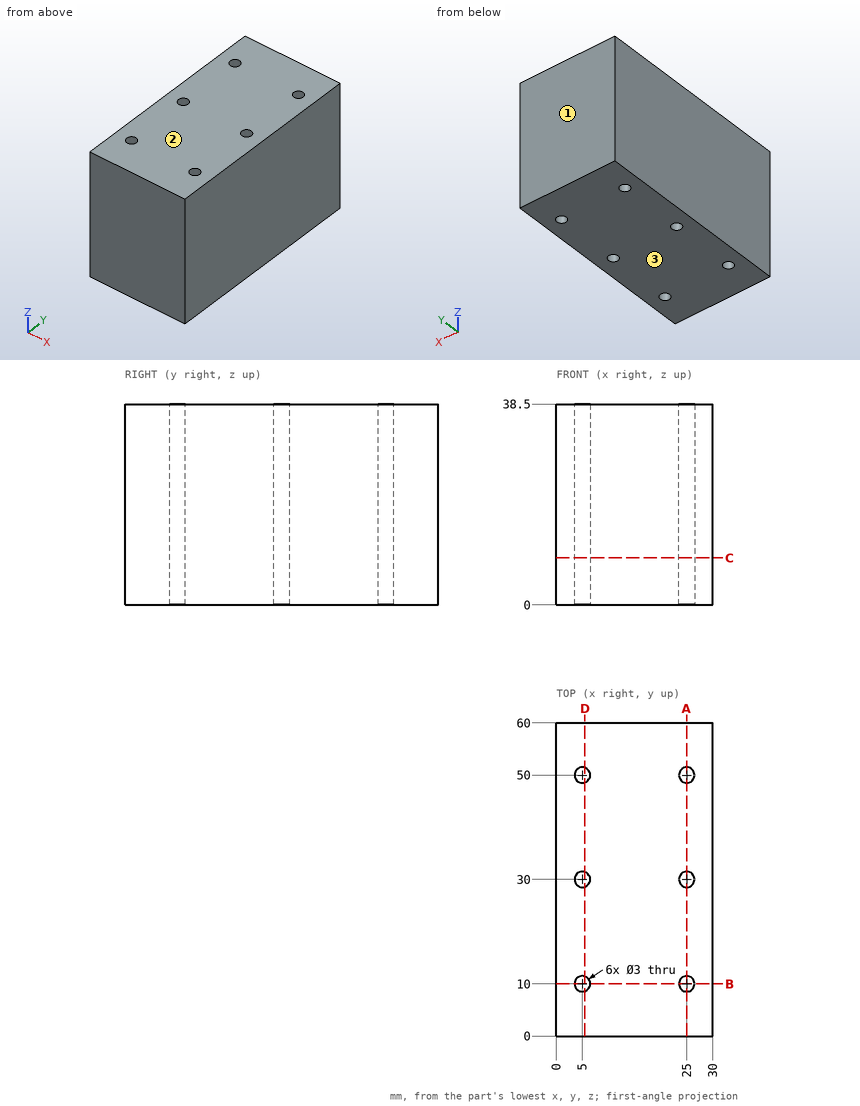
Can you work these out from the drawing? Everything is in mm from the part's minimum corner. Give positions to 0.01 mm unless a question says otherwise; leave off trailing zeros. Order: outer loops, then holes, each group sorted by start corner. A loop starts at its lowest first (then second) coordinate and runs counter-clockwise, first axis right, second up. Notation, with made-up numbers: M 30.25,8.5 L 88.25,8.5 A12 cw 88.25,25.5 Z; hole C -6.75,27.25 d9. An arc over 180 degrees is marked long. One line per question, with ' | ' between items.
1. I want a section at A-A (x = 25). List the corners of the cut face in (y, z) for me, and give its area (3 significant figures).
Results:
outline: M 0,0 L 8.5,0 L 8.5,38.5 L 0,38.5 Z; M 11.5,0 L 28.5,0 L 28.5,38.5 L 11.5,38.5 Z; M 31.5,0 L 48.5,0 L 48.5,38.5 L 31.5,38.5 Z; M 51.5,0 L 60,0 L 60,38.5 L 51.5,38.5 Z | area: 1,960 mm²
2. I want a section at D-D (x = 5.5). List the corners of the cut face in (y, z) for me.
Results:
outline: M 0,0 L 8.59,0 L 8.59,38.5 L 0,38.5 Z; M 11.41,0 L 28.59,0 L 28.59,38.5 L 11.41,38.5 Z; M 31.41,0 L 48.59,0 L 48.59,38.5 L 31.41,38.5 Z; M 51.41,0 L 60,0 L 60,38.5 L 51.41,38.5 Z
3. I want a section at C-C (z = 9). List the corners of the cut face in (x, y) for me, and give its area (3 significant figures).
Results:
outline: M 0,0 L 30,0 L 30,60 L 0,60 Z; hole C 5,10 d3; hole C 5,30 d3; hole C 5,50 d3; hole C 25,10 d3; hole C 25,30 d3; hole C 25,50 d3 | area: 1,760 mm²
4. If I drill on line 1 (Y direction, x = 5, z = 27); line 2 (X direction, y = 31, z = 29); line 3 (Y direction, x = 6.25, z = 3), over which ranges is the centre line in solid material (lowest first)?
Results:
line 1: 0 to 8.5, 11.5 to 28.5, 31.5 to 48.5, 51.5 to 60 | line 2: 0 to 3.88, 6.12 to 23.88, 26.12 to 30 | line 3: 0 to 9.17, 10.83 to 29.17, 30.83 to 49.17, 50.83 to 60
5. I'm going to push a flat-ended pin straight in: pin 1 (2.5 mm diameter, centred on x = 25, y = 30, fed in from +Z). Where does the tip first touch, or does it pass through?
Results:
pin 1: through
6. We'd pull the mould along Z, two halves only. Please class the marked faces 1, 2 and 3: +Z half, -Z half, draft (parallel to the pull), parting line (faces both ways), or undercut.
Results:
face 1: draft | face 2: +Z half | face 3: -Z half
7. I want a section at B-B (y = 10). List the corners of the cut face in (x, z) for me, and give its area (3 significant figures).
Results:
outline: M 0,0 L 3.5,0 L 3.5,38.5 L 0,38.5 Z; M 6.5,0 L 23.5,0 L 23.5,38.5 L 6.5,38.5 Z; M 26.5,0 L 30,0 L 30,38.5 L 26.5,38.5 Z | area: 924 mm²
